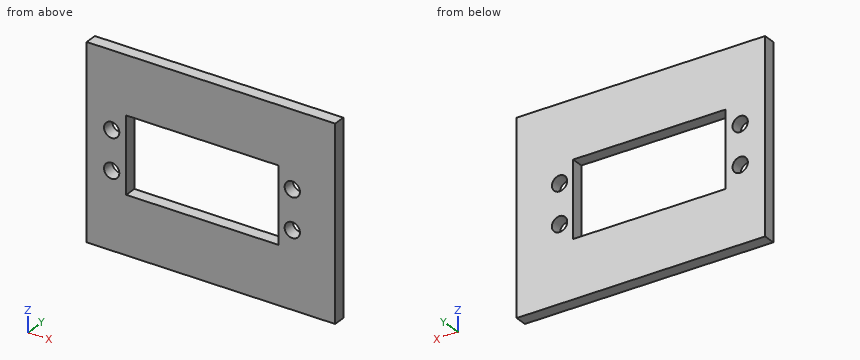
Autodesk Inventor part; units mm, degrees
ref_plane "YZ Plane" through (0, 0, 0) normal (1, 0, 0) x (0, 1, 0)
ref_plane "XZ Plane" through (0, 0, 0) normal (0, 1, 0) x (-1, 0, 0)
ref_plane "XY Plane" through (0, 0, 0) normal (0, 0, 1) x (1, 0, 0)
sketch "Sketch1" plane through (0, 0, 0) normal (0, 1, 0) x (-1, 0, 0)
  circle A0 centre (-33.79, -5.085) radius 2
  circle A1 centre (-33.79, 5.085) radius 2
  circle A2 centre (13.47, -5.085) radius 2
  circle A3 centre (13.47, 5.085) radius 2
  line L0 (20, 25) -> (-45, 25)
  line L1 (-45, 25) -> (-45, -25)
  line L2 (-45, -25) -> (20, -25)
  line L3 (20, -25) -> (20, 25)
  line L4 (9.66, 9.91) -> (-30.22, 9.91)
  line L5 (-30.22, 9.91) -> (-30.22, -9.91)
  line L6 (-30.22, -9.91) -> (9.66, -9.91)
  line L7 (9.66, -9.91) -> (9.66, 9.91)
  point P0 (0, 0)
  point P1 (0, 0)
  dimension "d0" = 4
  dimension "d1" = 4
  dimension "d2" = 4
  dimension "d3" = 4
  dimension "d4" = 13.47
  dimension "d5" = 5.085
  dimension "d6" = 10.17
  dimension "d7" = 13.47
  dimension "d8" = 33.79
  dimension "d9" = 5.085
  dimension "d10" = 10.17
  dimension "d12" = 50
  dimension "d13" = 65
  dimension "d15" = 25
  dimension "d25" = 9.66
  dimension "d26" = 19.82
  dimension "d27" = 9.91
  dimension "d28" = 39.88
  dimension "d29" = 33.79
  dimension "d30" = 20
extrude "Extrusion1" add sketch "Sketch1" along normal blind 3.18
properties part number "Hombro_servo"
Design review of the part built by this model. Coordinates are the model's own, in mm. Coordinates: 2 decimals unless noted, no trailing zeros. Loops run counter-clockwise (first coordinate to the right, second up) from the corner with the lowest first, then second, coordinate; pieces in that order, holes last. Notation, with made-up numbers: M 71.25,-3.5 L 76.25,-3.5 A17 cw 76.25,28.5 Z; hole C 43,47 d4. An arc over 180 degrees is marked long. Answer as CSV lines item,"result".
Item 1: For probe 1 along Z at (x, y) = (-13.47, 2.55) (3 decimals); probe 2 along X at (y, z) = (0.3, -5); probe 3 along X at (y, z) = (1.7, -8), list the stretches that pass through material, from the lowest coordinate up.
Answer list:
probe 1,"-25 to -7.085, -3.085 to 3.085, 7.085 to 25"
probe 2,"-20 to -15.47, -11.47 to -9.66, 30.22 to 31.79, 35.79 to 45"
probe 3,"-20 to -9.66, 30.22 to 45"
Item 2: Add section A-A on x = -13.47. State the section outline as (y, z) points (3 decimals), plus the area to 3 significant figures.
Answer list:
outline,"M 0,-25 L 3.18,-25 L 3.18,-7.085 L 0,-7.085 Z; M 0,-3.085 L 3.18,-3.085 L 3.18,3.085 L 0,3.085 Z; M 0,7.085 L 3.18,7.085 L 3.18,25 L 0,25 Z"
area,"134 mm²"
Item 3: Add section D-D on y = 2.2. State the section outline as (x, z) points (3 decimals), plus the area to 3 significant figures.
Answer list:
outline,"M -20,-25 L 45,-25 L 45,25 L -20,25 Z; hole C -13.47,-5.085 d4; hole C -13.47,5.085 d4; hole M -9.66,-9.91 L 30.22,-9.91 L 30.22,9.91 L -9.66,9.91 Z; hole C 33.79,-5.085 d4; hole C 33.79,5.085 d4"
area,"2,410 mm²"
Item 4: For P1, Ø5, axis at x = -13.47, z = 5.085, coming from the -Y side, flat-tipped, find the tip position at first contact; note if it passes through.
Answer list:
P1,"y = 0"
Item 5: Add section B-B on z = 2. State the section outline as (x, y) points, plus the area to 3 significant figures.
Answer list:
outline,"M -20,0 L -9.66,0 L -9.66,3.18 L -20,3.18 Z; M 30.22,0 L 45,0 L 45,3.18 L 30.22,3.18 Z"
area,"79.9 mm²"
Item 6: Add section C-C on x = -6. State the section outline as (y, z) points, plus the area to 3 significant figures.
Answer list:
outline,"M 0,-25 L 3.18,-25 L 3.18,-9.91 L 0,-9.91 Z; M 0,9.91 L 3.18,9.91 L 3.18,25 L 0,25 Z"
area,"96.0 mm²"
